Design review of the part built by this model. Coordinates are the model's own, in mm. Round coordinates to 2 decimals unless told otherwise and drop trailing zeros. Loops run counter-clockwise (first coordinate to the right, second up) from the corner with the lowest first, then second, coordinate; pieces in that order, holes last. Notation, with made-up numbers: M -39.75,-6 L -31.75,-6 A8 ccw -31.75,4 Z; hole C 55.25,21 d9. An arc over 180 degrees is marked long. Use a Markdown table: item, result.
from build123d import *

# Parameters (mm, degrees)
ESBO_O1_W                = 88.020382005
ESBO_O1_H                = 5.5
ESBO_O1_W_2              = 3
ESBO_O1_H_2              = 90.38122327
RESSALTO_EXTRUS_O1_DEPTH = 3


with BuildPart() as part:
    # Esboço1 → Ressalto-extrusão1 (new body)
    with BuildSketch(Plane.XY):
        Polygon((-308.071337018, 0), (-308.071337018, -3), (-220.050955012, -3), (-220.050955012, 0), (-132.031337017, 0), (-132.031337017, -3), (-44.010955012, -3), (-44.010955012, 0), (0, 0), (0, 180.76244654), (-44.010191002, 180.76244654), (-44.010191002, 186.26244654), (0, 186.26244654), (0, 397), (-352.08152802, 397), (-352.08152802, 186.26244654), (-308.071337018, 186.26244654), (-308.071337017, 180.76244654), (-352.08152802, 180.76244654), (-352.08152802, 0), align=None)
        with Locations((-176.04076401, 183.51244654)):
            Rectangle(ESBO_O1_W, ESBO_O1_H, mode=Mode.SUBTRACT)
        with Locations((-176.04076401, 90.38122327)):
            Rectangle(ESBO_O1_W_2, ESBO_O1_H_2, mode=Mode.SUBTRACT)
    extrude(amount=RESSALTO_EXTRUS_O1_DEPTH)


solid = part.part
1. Take a section at A-A on x = -39. Give the boundary of the cut face in (y, z).
Check values:
| item | result |
|---|---|
| outline | M 0,0 L 180.76,0 L 180.76,3 L 0,3 Z; M 186.26,0 L 397,0 L 397,3 L 186.26,3 Z |
2. Insertion check: pin 1 (0.9 mm diameter, centred on x = -179, z = 1, fed in from -Y); pin 2 (5 mm diameter, centred on x = -311, y = 347, fed in from -Z); pin 3 (1.5 mm diameter, centred on y = -1, z = 1.5, fed in from -X); pin 4 (1.5 mm diameter, centred on y = -2, z = 1, fed in from +X). Each pin has a flat end and moves straight along its axis. Give the tip position at first contact, or say it passes through.
Check values:
| item | result |
|---|---|
| pin 1 | stops at y = 0 |
| pin 2 | stops at z = 0 |
| pin 3 | stops at x = -308.07 |
| pin 4 | stops at x = -44.01 |
3. Wall thickness on line 1 along Y through (x, z) = (-136, 0.45); line 2 along X through (y, z) = (61, 0.7): over which ranges is each line inside the solid? List them lowest first. Write a range as from..to.
Check values:
| item | result |
|---|---|
| line 1 | y = 0..180.76, 186.26..397 |
| line 2 | x = -352.08..-177.54, -174.54..0 |
